```python
from build123d import *
from build123d.topology import SkipClean

# Parameters (mm, degrees)
BOSS_EXTRUDE4_DEPTH             = 70
F_1_0MM_DOWEL_HOLE1_D           = 30
SKETCH4_R                       = 25
SKETCH4_R_2                     = 15
BOSS_EXTRUDE5_DEPTH             = 5
CUT_EXTRUDE4_DEPTH              = 499.121471129
CUT_EXTRUDE4_DEPTH_BACK         = 499.121471129
CUT_EXTRUDE5_DEPTH              = 55
F_10_0MM_DOWEL_HOLE1_AT_2_COUNT = 2
F_10_0MM_DOWEL_HOLE1_AT_2_PITCH = 155.724133524
F_10_0MM_DOWEL_HOLE1_AT_3_COUNT = 2
F_10_0MM_DOWEL_HOLE1_AT_3_PITCH = 183.115416505
CUT_EXTRUDE6_START              = -158.910746
SKETCH22_R                      = 40
CUT_EXTRUDE6_DEPTH              = 146.370732


with BuildPart() as part:
    # Sketch2 → Boss-Extrude4 (new, symmetric)
    with BuildSketch(Plane.XY):
        with BuildLine():
            Line((-200, 0), (200, 0))
            Line((200, 0), (200, 250))
            ThreePointArc((200, 250), (0, 450), (-200, 250))
            Line((-200, 250), (-200, 0))
        make_face()
    extrude(amount=BOSS_EXTRUDE4_DEPTH, both=True)

    # 1.0mm Dowel Hole1 (through all)
    with Locations(Plane(origin=(0, 250, 70), x_dir=(1, 0, 0), z_dir=(0, 0, 1))):
        with Locations((0, 0)):
            Hole(F_1_0MM_DOWEL_HOLE1_D / 2)

    # Sketch4 → Boss-Extrude5 (add)
    with SkipClean():  # the faces are left unmerged after this step: merging them gives an invalid solid
        with BuildSketch(Plane.XY.offset(70)):
            with Locations((0, 250)):
                Circle(SKETCH4_R)
            with Locations((0, 250)):
                Circle(SKETCH4_R_2, mode=Mode.SUBTRACT)
        extrude(amount=BOSS_EXTRUDE5_DEPTH)
    add(part.part.scale(1), mode=Mode.REPLACE)  # the faces are merged on a copy

    # Sketch13 → Cut-Extrude4 (cut, two sides: drawn at the far end of the back side and taken through both)
    with BuildSketch(Plane(origin=(0, 0, 0), x_dir=(0, 0, -1), z_dir=(1, 0, 0)).offset(-CUT_EXTRUDE4_DEPTH_BACK)):
        Polygon((0, -922.414379545), (0, 0), (0, 450), (0, 1372.414379545), (1844.828759089, 1372.414379545), (1844.828759089, -922.414379545), align=None)
    extrude(amount=CUT_EXTRUDE4_DEPTH + CUT_EXTRUDE4_DEPTH_BACK, mode=Mode.SUBTRACT)

    # Sketch14 → Cut-Extrude5 (cut)
    with BuildSketch(Plane(origin=(0, 0, 0), x_dir=(-1, 0, 0), z_dir=(0, 0, -1))):
        with BuildLine():
            Line((-185, 45), (-185, 200))
            ThreePointArc((-185, 200), (-182.128554255, 215.817234791), (-173.880670381, 229.615877068))
            Line((-173.880670381, 229.615877068), (-88.466194885, 327.330345677))
            ThreePointArc((-88.466194885, 327.330345677), (-70.735263863, 343.823091221), (-49.999974949, 356.330863371))
            Line((-49.999974949, 356.330863371), (-49.999974949, 420.000023858))
            ThreePointArc((-49.999974949, 420.000023858), (0, 440), (49.999974949, 420.000023858))
            Line((49.999974949, 420.000023858), (49.999974949, 356.330863371))
            ThreePointArc((49.999974949, 356.330863371), (70.735263863, 343.823091221), (88.466194885, 327.330345677))
            Line((88.466194885, 327.330345677), (173.880670381, 229.615877068))
            ThreePointArc((173.880670381, 229.615877068), (182.128554255, 215.817234791), (185, 200))
            Line((185, 200), (185, 45))
            Line((185, 45), (178.301270189, 20))
            Line((178.301270189, 20), (178.301270189, 0))
            Line((178.301270189, 0), (-178.301270189, 0))
            Line((-178.301270189, 0), (-178.301270189, 20))
            Line((-178.301270189, 20), (-185, 45))
        make_face()
    extrude(amount=-CUT_EXTRUDE5_DEPTH, mode=Mode.SUBTRACT)

    # Sketch18 → M8x1.0 Tapped Hole1 (revolve, cut)
    with BuildSketch(Plane(origin=(-200, 15, 25), x_dir=(0, 0, 1), z_dir=(0, 1, 0))):
        Polygon((0, 0), (0, 13.103012167), (3.5, 11), (3.5, 0), align=None)
    m8x1_0_tapped_hole1 = revolve(axis=Axis((-206.35, 15, 25), (1, 0, 0)), mode=Mode.SUBTRACT)

    # Mirror2: M8x1.0 Tapped Hole1 across plane
    add(m8x1_0_tapped_hole1.mirror(Plane(origin=(0, 0, 0), x_dir=(0, 0, 1), z_dir=(1, 0, 0))), mode=Mode.SUBTRACT)

    # Sketch21 → 10.0mm Dowel Hole1 (revolve, cut)
    with BuildSketch(Plane(origin=(185, 265, 0), x_dir=(0, 1, 0), z_dir=(1, 0, 0))):
        Polygon((0, 0), (0, 50), (5, 45), (5, 0), align=None)
    f_10_0mm_dowel_hole1 = revolve(axis=Axis((185, 265, -6.35), (0, 0, 1)), mode=Mode.SUBTRACT)

    # 10.0mm Dowel Hole1 at 2: 10.0mm Dowel Hole1 ×2
    with Locations(*[Vector(-0.7384855670659363, 0.6742692839180076, 0) * (i * F_10_0MM_DOWEL_HOLE1_AT_2_PITCH) for i in range(1, F_10_0MM_DOWEL_HOLE1_AT_2_COUNT)]):
        add(f_10_0mm_dowel_hole1, mode=Mode.SUBTRACT)

    # 10.0mm Dowel Hole1 at 3: 10.0mm Dowel Hole1 ×2
    with Locations(*[Vector(-0.6280193511079233, 0.7781977220693871, 0) * (i * F_10_0MM_DOWEL_HOLE1_AT_3_PITCH) for i in range(1, F_10_0MM_DOWEL_HOLE1_AT_3_COUNT)]):
        add(f_10_0mm_dowel_hole1, mode=Mode.SUBTRACT)

    # Mirror3: 10.0mm Dowel Hole1 across plane
    add(f_10_0mm_dowel_hole1.mirror(Plane(origin=(0, 0, 0), x_dir=(0, 0, 1), z_dir=(1, 0, 0))), mode=Mode.SUBTRACT)

    # Mirror3 copy 1 sketch → Mirror3 copy 1 (revolve, cut)
    with BuildSketch(Plane(origin=(-69.999974949, 370, 0), x_dir=(0, 1, 0), z_dir=(-1, 0, 0))):
        Polygon((0, 0), (0, -50), (5, -45), (5, 0), align=None)
    revolve(axis=Axis((-69.999974949, 370, -6.35), (0, 0, -1)), mode=Mode.SUBTRACT)

    # Mirror3 copy 2 sketch → Mirror3 copy 2 (revolve, cut)
    with BuildSketch(Plane(origin=(-69.999974949, 407.5, 0), x_dir=(0, 1, 0), z_dir=(-1, 0, 0))):
        Polygon((0, 0), (0, -50), (5, -45), (5, 0), align=None)
    revolve(axis=Axis((-69.999974949, 407.5, -6.35), (0, 0, -1)), mode=Mode.SUBTRACT)

    # Sketch22 → Cut-Extrude6 (cut)
    with BuildSketch(Plane(origin=(-114.263809021, 426.438340731, 0), x_dir=(0, 0, -1), z_dir=(-0.25881904510252135, 0.9659258262890681, 0)).offset(CUT_EXTRUDE6_START)):
        with Locations((0, 45)):
            Circle(SKETCH22_R)
    cut_extrude6 = extrude(amount=CUT_EXTRUDE6_DEPTH, mode=Mode.SUBTRACT)

    # Mirror4: Cut-Extrude6 across plane
    add(cut_extrude6.mirror(Plane(origin=(0, 0, 0), x_dir=(0, 0, 1), z_dir=(1, 0, 0))), mode=Mode.SUBTRACT)


solid = part.part
```
Build history of the part. All positions in model axes, mm. A direction names the side the tool comes from. Round coordinates to 2 decimals unless told otherwise and drop trailing zeros. Loops run counter-clockwise (first coordinate to the right, second up) from the corner with the lowest first, then second, coordinate; pieces in that order, holes last.
Item 1: Which spindle directions (+Z, -Z, +X, -X, +Y, -Y) get a long thin tool onto all of the face, cutting with end or side? Do faces 4 (the face through (4.4, 449.95, 43.27)), 5 (the face through (178.301, 10, 27)), 6 (the face through (-68.5, 412.27, 22.18)). Say none if no direction does.
Item 2: Saw through at A-A (x = 0). List the corners of the cut face in (y, z).
Item 3: Drill centre lines: line 1 along X through (y, z) = (250, 60); line 2 along X through (y, z) = (66, 35.5); line 3 along X through (y, z) = (265, 21). Where is each one in solid material? Low to high.
Item 4: Two-plate mould, pull along Y, no slides. Class faces 1 (the face through (-53, 402, 0)), 2 (the face through (-70.5, 344, 27.1)), 3 (the face through (182.208, 215.605, 27.115)): released by +Y, released by -Y, zero draft, split by the parting line, or undercut.
Item 5: Saw through at B-B (z = 34). State how many separate pieces and enclosed holes the cut face has, then the cut area to 3 significant figures.
Item 6: Pin check, flat tips, straight feed: P1, Ø1, axis at x = -55, z = 21, coming from the -Y side; P2, Ø9, axis at x = -70, y = 370, coming from the +Z side; P3, Ø6.5, axis at y = 15, z = 25, coming from the -X side. Stop position of each tip, or through.
Worked answers:
1. face 4: +Z, -Z, +Y
1. face 5: -Z, -Y
1. face 6: -Z
2. outline: (0, 55) - (235, 55) - (235, 75) - (225, 75) - (225, 70) - (0, 70) - close; (265, 55) - (440, 55) - (440, 0) - (450, 0) - (450, 70) - (275, 70) - (275, 75) - (265, 75) - close
3. line 1: x = -200 to -15, 15 to 200
3. line 2: x = -200 to -185, 185 to 200
3. line 3: x = -199.44 to -190, -180 to -152.84, 152.84 to 180, 190 to 199.44
4. face 1: zero draft
4. face 2: released by -Y
4. face 3: undercut
5. separate pieces: 3
5. enclosed holes: 6
5. area: 32,200 mm2
6. P1: stops at y = 353.57
6. P2: stops at z = 70
6. P3: stops at x = -188.85
